For this review, take the finished solid that the model builds, in its own axes (mm). A direction names the side the tool comes from. Give positions to 0.01 mm unless a question says otherwise; leave off trailing zeros. Loops run counter-clockwise (first coordinate to the right, second up) from the corner with the lowest first, then second, coordinate; pieces in that order, holes last.
```python
from build123d import *

# Parameters (mm, degrees)
SKETCH1_W           = 50
SKETCH1_H           = 50
BOSS_EXTRUDE1_DEPTH = 4
SKETCH2_W           = 4
SKETCH2_H           = 50
BOSS_EXTRUDE2_DEPTH = 45
SKETCH4_R           = 6
BOSS_EXTRUDE3_DEPTH = 40
SKETCH5_R           = 3.25
CUT_EXTRUDE1_DEPTH  = 40


with BuildPart() as part:
    # Sketch1 → Boss-Extrude1 (new body)
    with BuildSketch(Plane.XY):
        Rectangle(SKETCH1_W, SKETCH1_H)
    extrude(amount=BOSS_EXTRUDE1_DEPTH)

    # Sketch2 → Boss-Extrude2 (add)
    with BuildSketch(Plane.XY.offset(4)):
        with Locations((-23, 0)):
            Rectangle(SKETCH2_W, SKETCH2_H)
    extrude(amount=BOSS_EXTRUDE2_DEPTH)

    # Sketch4 → Boss-Extrude3 (add)
    with BuildSketch(Plane(origin=(-21, 0, 0), x_dir=(0, 0, -1), z_dir=(1, 0, 0))):
        with Locations(Location((-20, 0, 0), (0, 0, 270))):
            Circle(SKETCH4_R)
    extrude(amount=BOSS_EXTRUDE3_DEPTH)

    # Sketch5 → Cut-Extrude1 (cut)
    with BuildSketch(Plane.XY.offset(4)):
        with Locations((20, 20)):
            Circle(SKETCH5_R)
        with Locations((20, -20)):
            Circle(SKETCH5_R)
    extrude(amount=-CUT_EXTRUDE1_DEPTH, mode=Mode.SUBTRACT)


solid = part.part
```
Q1. For probe 1 along Y at (x, z) = (20, 2.9); probe 2 along Z at (x, y) = (-12.5, 0); probe 3 along Z at (x, y) = (10.5, -10.5), list the stretches that pass through material, from the lowest coordinate up.
Answers:
probe 1: y = -25 to -23.25, -16.75 to 16.75, 23.25 to 25
probe 2: z = 0 to 4, 14 to 26
probe 3: z = 0 to 4
Q2. For pin 1 Ø13 at (y, z) = (2.5, 19.5) entering from +X; pin 2 Ø8.5 at (x, y) = (20, -20) entering from +Z; pin 3 Ø23 at (x, y) = (2, 5) entering from +Z; pin 4 Ø3 at (x, z) = (-8.5, 29) entering from +Y, all flat-tipped, find the tip position at first contact; note any pin that passes through.
Answers:
pin 1: stops at x = 19
pin 2: stops at z = 4
pin 3: stops at z = 26
pin 4: passes through
Q3. Consider section A-A on x = 20. Give the boundary of the cut face in (y, z).
Answers:
outline: (-25, 0) - (-23.25, 0) - (-23.25, 4) - (-25, 4) - close; (-16.75, 0) - (16.75, 0) - (16.75, 4) - (-16.75, 4) - close; (23.25, 0) - (25, 0) - (25, 4) - (23.25, 4) - close
Q4. Consider section C-C on y = 0. Give the boundary of the cut face in (x, z).
Answers:
outline: (-25, 0) - (25, 0) - (25, 4) - (-21, 4) - (-21, 14) - (19, 14) - (19, 26) - (-21, 26) - (-21, 49) - (-25, 49) - close
Q5. Mouldability with a two-part tool opening along Z and no side actions: class faces 4 (the flat face through (0, 0, 0)), 5 (the flat face through (25, 0, 2)), 6 (the flat face through (2, 0, 4)) as +Z half, -Z half, draft (parallel to the pull), parting line (faces both ways), or undercut.
Answers:
face 4: -Z half
face 5: draft
face 6: undercut
Q6. Consider section D-D on z = 5.5. Give the boundary of the cut face in (x, y).
Answers:
outline: (-25, -25) - (-21, -25) - (-21, 25) - (-25, 25) - close
Q7. Consider section B-B on y = 20. Give the boundary of the cut face in (x, z).
Answers:
outline: (-25, 0) - (16.75, 0) - (16.75, 4) - (-21, 4) - (-21, 49) - (-25, 49) - close; (23.25, 0) - (25, 0) - (25, 4) - (23.25, 4) - close
Q8. Machinability: for faces 1 (the cylindrical face through (-1.28, 0.78, 14.05)), 2 (the cylindrical face through (17.605, -17.803, 2.028)), 3 (the flat face through (19, 0, 20)), which of the approach directions +Z, -Z, +X, -X, +Y, -Y give a long, thin tool a straight path to every point of the face, cutting with its end or side? Answer none if there is none.
Answers:
face 1: +X
face 2: +Z, -Z
face 3: +Z, +X, +Y, -Y
